```python
from build123d import *

# Parameters (mm, degrees)
ESQUISSE1_R             = 20
BOSS_EXTRU_1_DEPTH      = 6
ESQUISSE2_R             = 5
ENL_V_MAT_EXTRU_1_DEPTH = 29.91366459
ESQUISSE3_R             = 1.393852397
ENL_V_MAT_EXTRU_2_DEPTH = 29.91366459
ENL_V_MAT_EXTRU_3_DEPTH = 29.91366459


with BuildPart() as part:
    # Esquisse1 → Boss.-Extru.1 (new body)
    with BuildSketch(Plane.XY):
        Circle(ESQUISSE1_R)
    extrude(amount=BOSS_EXTRU_1_DEPTH)

    # Esquisse2 → Enlèv. mat.-Extru.1 (cut, through all)
    with BuildSketch(Plane.XY.offset(6)):
        Circle(ESQUISSE2_R)
    extrude(amount=-ENL_V_MAT_EXTRU_1_DEPTH, mode=Mode.SUBTRACT)

    # Esquisse3 → Enlèv. mat.-Extru.2 (cut, through all)
    with BuildSketch(Plane.XY.offset(6)):
        with Locations((0, 6.5)):
            Circle(ESQUISSE3_R)
        with Locations((5.629165125, -3.25)):
            Circle(ESQUISSE3_R)
        with Locations((-5.629165125, -3.25)):
            Circle(ESQUISSE3_R)
    extrude(amount=-ENL_V_MAT_EXTRU_2_DEPTH, mode=Mode.SUBTRACT)

    # Esquisse4 → Enlèv. mat.-Extru.3 (cut, through all)
    with BuildSketch(Plane(origin=(0, 0, 0), x_dir=(-1, 0, 0), z_dir=(0, 0, -1))):
        with BuildLine():
            Line((5.2, 16.80000003), (5.2, 19.312172327))
            ThreePointArc((5.2, 19.312172327), (0, 20), (-5.2, 19.312172327))
            Line((-5.2, 19.312172327), (-5.2, 16.80000003))
            Line((-5.2, 16.80000003), (5.2, 16.80000003))
        make_face()
    extrude(amount=-ENL_V_MAT_EXTRU_3_DEPTH, mode=Mode.SUBTRACT)


solid = part.part
```
Model file for the job. Use its own axes, mm. A direction names the side the tool comes from. Coordinates: 2 decimals unless noted, no trailing zeros. Loops run counter-clockwise (first coordinate to the right, second up) from the corner with the lowest first, then second, coordinate; pieces in that order, holes last. Notation, with made-up numbers: (-32.5, 63) - (8.5, 63) arc R26 ccw to (8.5, 78) - close; hole circle Ø9 at (28, -29). An arc over 180 degrees is marked (long way). Write item = value, one per line. Start each with the question number.
Item 1: Drop flat-ended pins along their axis: pin 1 Ø10 at (x, y) = (-12.5, -10.5) entering from -Z; pin 2 Ø2 at (x, z) = (1.5, 3) entering from +Y; pin 3 Ø1 at (x, z) = (-13, 3.5) entering from +Y; pin 4 Ø0.8 at (y, z) = (18, 2) entering from -X. Give the stop position or say it passes through.
Item 2: Saw through at D-D, the plane y = 4. List the corners of the cut face in (x, z).
Item 3: Saw through at B-B, the plane z = 2.6. List the corners of the cut face in (x, y).
Item 4: Saw through at C-C, the plane y = 0. List the corners of the cut face in (x, z).
Item 5: Saw through at A-A, the plane x = 0. List the corners of the cut face in (y, z), then the cut area to 3 significant figures.
Item 6: Pull direction Y, two halves, no side cores. Call faces 1 (the face through (-0.806, -19.984, 2.958)), 2 (the face through (4, -4, 0)), 3 (the face through (6.92, -3.78, 3.04)), 4 (the face through (0, 16.8, 3)): +Y half, -Y half, draft (parallel to the pull), parting line (faces both ways), or undercut.
Item 7: Wall check: probe 1 along X at (y, z) = (-2, 3); probe 2 along X at (y, z) = (-3, 3.2); probe 3 along Y at (x, z) = (-1, 0.6). Give the ranges that are in metal, low to high. Write a range as [from, to].
Item 8: 3-axis set-ups, long thin cutter, end or side, ignore diameter. For faces 5 (the face through (-6.735, -4.098, 3.042)), 6 (the face through (5.2, 18, 3)): which of +Z, -Z, +X, -X, +Y, -Y reach the whole face in a straight line?
Answers:
q1.pin_1 = 0
q1.pin_2 = 16.8
q1.pin_3 = 15.61
q1.pin_4 = -9.5
q2.outline = (-19.6, 0) - (-3, 0) - (-3, 6) - (-19.6, 6) - close; (3, 0) - (19.6, 0) - (19.6, 6) - (3, 6) - close
q3.outline = (-5.2, 16.8) - (-5.2, 19.31) arc R20 ccw (long way) to (5.2, 19.31) - (5.2, 16.8) - close; hole circle Ø2.79 at (-5.63, -3.25); hole circle Ø10 at (0, 0); hole circle Ø2.79 at (0, 6.5); hole circle Ø2.79 at (5.63, -3.25)
q4.outline = (-20, 0) - (-5, 0) - (-5, 6) - (-20, 6) - close; (5, 0) - (20, 0) - (20, 6) - (5, 6) - close
q5.outline = (-20, 0) - (-5, 0) - (-5, 6) - (-20, 6) - close; (5, 0) - (5.11, 0) - (5.11, 6) - (5, 6) - close; (7.89, 0) - (16.8, 0) - (16.8, 6) - (7.89, 6) - close
q5.area = 144 mm2
q6.face_1 = parting line
q6.face_2 = draft
q6.face_3 = undercut
q6.face_4 = +Y half
q7.probe_1 = [-19.9, -6.25], [-5.01, -4.58], [4.58, 5.01], [6.25, 19.9]
q7.probe_2 = [-19.77, -7], [-4.26, -4], [4, 4.26], [7, 19.77]
q7.probe_3 = [-19.97, -4.9], [4.9, 5.53], [7.47, 16.8]
q8.face_5 = +Z, -Z
q8.face_6 = +Z, -Z, +Y
